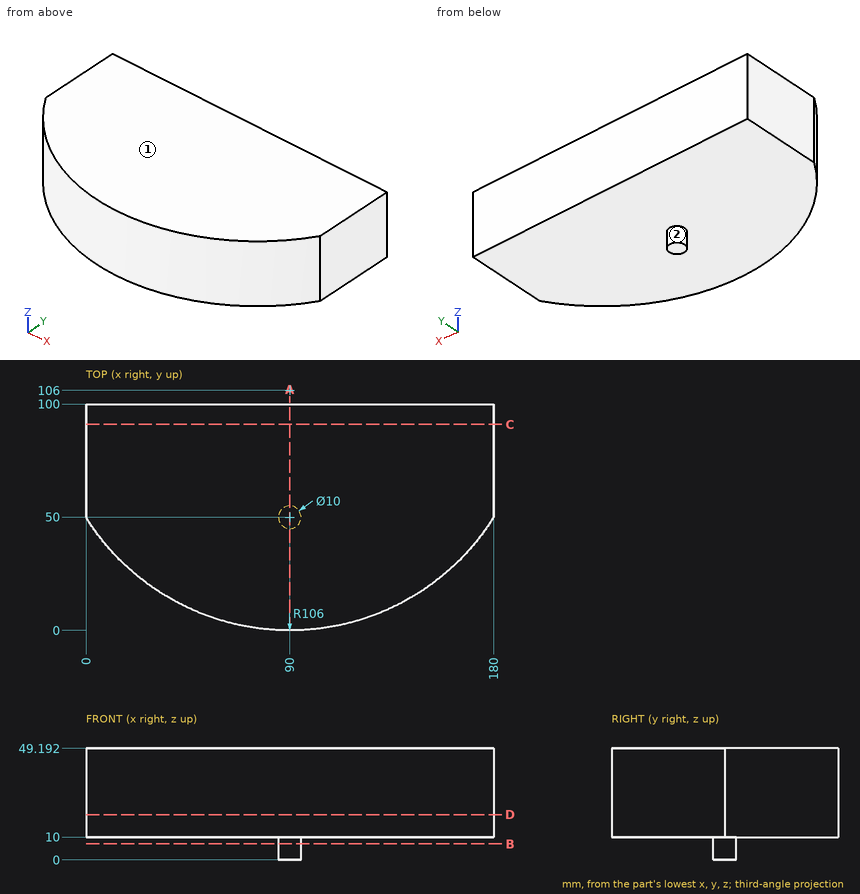
Check sheet for the drawn part. Datum: minimum x, y, z corner. Units: mm. A direction names the side the tool comes from. Round coordinates to 2 decimals unless told otherwise and drop trailing zeros. Order: outer loops, then holes, each group sorted by start corner. A loop starts at its lowest first (then second) coordinate and runs counter-clockwise, first axis right, second up.
(1) Access from +Z, -Z, +X, -X, +Y, -Y to the whole of each face (thin tool, end or side, straight path). Record for the marked faces 1 and 2.
(2) Scan lines: probe 1 along Z at (x, y) = (94, 45.5); probe 2 along X at (y, z) = (23.5, 43.5) (1 decimal); probe 3 along Y at (x, z) = (131, 12). Record each from-to range of solid material in increasing order.
(3) Cross-section at B-B, the plane z = 7. Enter the section's corners in (x, y).
(4) Go/stop test with flat-tipped pins: P1, Ø5, axis at x = 149, z = 31.5, coming from the -Y side; P2, Ø4, axis at x = 66.5, y = 33, coming from the -Z side; P3, Ø3, axis at x = 95.5, z = 7, coming from the +Y side. Record where each tip stops, or that it passes through.
(5) Cross-section at A-A, the plane x = 90. Enter the section's corners in (y, z), and give its area (3 significant figures).
(6) Cross-section at C-C, the plane y = 91. Enter the section's corners in (x, z).
(7) Cross-section at D-D, the plane z = 20. Enter the section's corners in (x, y).
Check sheet entries:
1. face 1: +Z, +X, -X, +Y, -Y
1. face 2: -Z
2. probe 1: z = 10 to 49.19
2. probe 2: x = 23.4 to 156.6
2. probe 3: y = 8.25 to 100
3. outline: circle Ø10 at (90, 50)
4. P1: stops at y = 16.31
4. P2: stops at z = 10
4. P3: stops at y = 53
5. outline: (0, 10) - (45, 10) - (45, 0) - (55, 0) - (55, 10) - (100, 10) - (100, 49.19) - (0, 49.19) - close
5. area: 4,020 mm2
6. outline: (0, 10) - (180, 10) - (180, 49.19) - (0, 49.19) - close
7. outline: (0, 50) arc R106 ccw to (180, 50) - (180, 100) - (0, 100) - close
